Work out the finished part from the listing and answer in its coordinate system (mm). Round coordinates to 2 decimals unless told otherwise and drop trailing zeros. Loops run counter-clockwise (first coordinate to the right, second up) from the corner with the lowest first, then second, coordinate; pieces in that order, holes last.
from build123d import *

# Parameters (mm, degrees)
SKETCH2_W           = 80
SKETCH2_H           = 80
BOSS_EXTRUDE1_DEPTH = 3
SKETCH3_R           = 2.15
SKETCH3_W           = 20
SKETCH3_H           = 40
CUT_EXTRUDE1_DEPTH  = 3
SKETCH4_W           = 5
SKETCH4_H           = 80
CUT_EXTRUDE2_DEPTH  = 10
SKETCH5_R           = 2
CUT_EXTRUDE3_DEPTH  = 10


with BuildPart() as part:
    # Sketch2 → Boss-Extrude1 (new body)
    with BuildSketch(Plane(origin=(0, 0, 0), x_dir=(1, 0, 0), z_dir=(0, 1, 0))):
        Rectangle(SKETCH2_W, SKETCH2_H)
    extrude(amount=BOSS_EXTRUDE1_DEPTH)

    # Sketch3 → Cut-Extrude1 (cut)
    with BuildSketch(Plane(origin=(0, 3, 0), x_dir=(1, 0, 0), z_dir=(0, 1, 0))):
        with Locations(Location((-29.845, 34.49, 0), (0, 0, 270))):
            Circle(SKETCH3_R)
        with Locations(Location((-19.975, 34.49, 0), (0, 0, 270))):
            Circle(SKETCH3_R)
        with Locations(Location((-19.975, -14.81, 0), (0, 0, 270))):
            Circle(SKETCH3_R)
        with Locations(Location((-29.845, -14.81, 0), (0, 0, 270))):
            Circle(SKETCH3_R)
        with Locations((-25, 10)):
            Rectangle(SKETCH3_W, SKETCH3_H)
    extrude(amount=-CUT_EXTRUDE1_DEPTH, mode=Mode.SUBTRACT)

    # Sketch4 → Cut-Extrude2 (cut)
    with BuildSketch(Plane(origin=(0, 3, 0), x_dir=(1, 0, 0), z_dir=(0, 1, 0))):
        with Locations((37.5, 0)):
            Rectangle(SKETCH4_W, SKETCH4_H)
    extrude(amount=-CUT_EXTRUDE2_DEPTH, mode=Mode.SUBTRACT)

    # Sketch5 → Cut-Extrude3 (cut)
    with BuildSketch(Plane.XZ):
        with Locations(Location((25, 0, 0), (0, 0, 270))):
            Circle(SKETCH5_R)
        with Locations(Location((-5, 0, 0), (0, 0, 270))):
            Circle(SKETCH5_R)
        with Locations(Location((-5, 30, 0), (0, 0, 270))):
            Circle(SKETCH5_R)
        with Locations(Location((25, 30, 0), (0, 0, 270))):
            Circle(SKETCH5_R)
    extrude(amount=-CUT_EXTRUDE3_DEPTH, mode=Mode.SUBTRACT)


solid = part.part
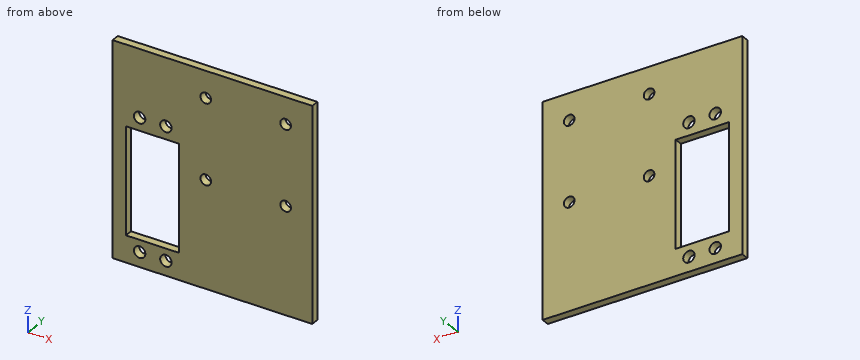
Item 1: Section C-C, the plane x = 25 is taken. Give the vertices of the cut face in (y, z).
Item 2: Section A-A, the plane x = -33.5 is taken. Give the vertices of the cut face in (y, z).
Item 3: Straight lines are drawn through the part: line 1 (X direction, y = 1.1, z = -34.49) (3 decimals); line 2 (X direction, y = 1.5, z = 30); line 3 (X direction, y = 0.7, z = 0). For each, find the intervals that lie inside material, in ascending order.
Item 4: Section D-D, the plane y = 2.3 is taken. State how many separate pieces and enclosed holes the cut face has, plus the area to 3 significant figures.
Item 5: Section B-B, the plane z = -34.49 is taken. Give the vertices of the cut face in (x, y) (3 decimals), plus the area to 3 significant figures.
Item 6: This flat-tipped pin is pushed along its axis until it touches: P1, Ø5, axis at x = -29.845, z = 14.81, coming from the +Y side. Where does it stop, or does it pass through?
Answer below:
1. outline: (0, -40) - (3, -40) - (3, -2) - (0, -2) - close; (0, 2) - (3, 2) - (3, 28) - (0, 28) - close; (0, 32) - (3, 32) - (3, 40) - (0, 40) - close
2. outline: (0, -40) - (3, -40) - (3, -30) - (0, -30) - close; (0, 10) - (3, 10) - (3, 40) - (0, 40) - close
3. line 1: x = -40 to -31.995, -27.695 to -22.125, -17.825 to 35
3. line 2: x = -40 to -7, -3 to 23, 27 to 35
3. line 3: x = -40 to -35, -15 to -7, -3 to 23, 27 to 35
4. separate pieces: 1
4. enclosed holes: 9
4. area: 5,090 mm2
5. outline: (-40, 0) - (-31.995, 0) - (-31.995, 3) - (-40, 3) - close; (-27.695, 0) - (-22.125, 0) - (-22.125, 3) - (-27.695, 3) - close; (-17.825, 0) - (35, 0) - (35, 3) - (-17.825, 3) - close
5. area: 199 mm2
6. P1: stops at y = 3
